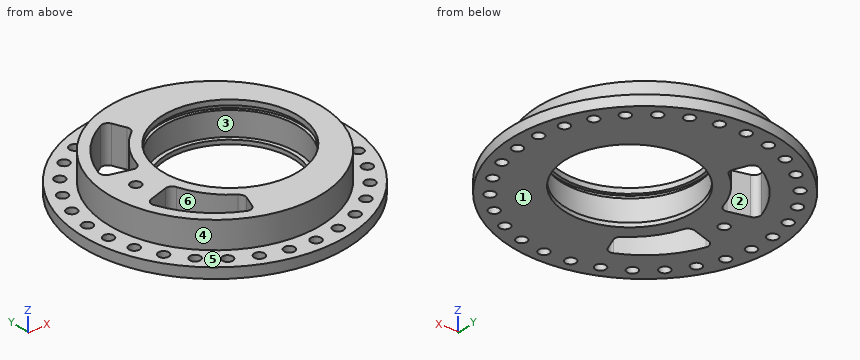
```python
from build123d import *

# Parameters (mm, degrees)
SKETCH1_R           = 63.5
BOSS_EXTRUDE1_DEPTH = 5
SKETCH2_R           = 51
BOSS_EXTRUDE2_DEPTH = 13
SKETCH3_R           = 32.5
CUT_EXTRUDE1_DEPTH  = 19
CUT_EXTRUDE9_START  = -2.5
SKETCH4_R           = 34
SKETCH4_R_2         = 32.5
CUT_EXTRUDE9_DEPTH  = 2
SKETCH6_R           = 32.5
SKETCH6_R_2         = 30.5
BOSS_EXTRUDE3_DEPTH = 2
SKETCH7_R           = 2.5
CUT_EXTRUDE10_DEPTH = 19
SKETCH9_R           = 2.5
CUT_EXTRUDE11_DEPTH = 19
CUT_EXTRUDE12_DEPTH = 19
FILLET1_R           = 3


with BuildPart() as part:
    # Sketch1 → Boss-Extrude1 (new body)
    with BuildSketch(Plane.XY):
        Circle(SKETCH1_R)
    extrude(amount=BOSS_EXTRUDE1_DEPTH)

    # Sketch2 → Boss-Extrude2 (add)
    with BuildSketch(Plane.XY.offset(5)):
        Circle(SKETCH2_R)
    extrude(amount=BOSS_EXTRUDE2_DEPTH)

    # Sketch3 → Cut-Extrude1 (cut, through all)
    with BuildSketch(Plane.XY.offset(18)):
        with Locations((7.5, 0)):
            Circle(SKETCH3_R)
    extrude(amount=-CUT_EXTRUDE1_DEPTH, mode=Mode.SUBTRACT)

    # Sketch4 → Cut-Extrude9 (cut)
    with BuildSketch(Plane.XY.offset(18).offset(CUT_EXTRUDE9_START)):
        with Locations((7.5, 0)):
            Circle(SKETCH4_R)
        with Locations((7.5, 0)):
            Circle(SKETCH4_R_2, mode=Mode.SUBTRACT)
    extrude(amount=-CUT_EXTRUDE9_DEPTH, mode=Mode.SUBTRACT)

    # Sketch6 → Boss-Extrude3 (add)
    with BuildSketch(Plane(origin=(0, 0, 0), x_dir=(-1, 0, 0), z_dir=(0, 0, -1))):
        with Locations((-7.5, 0)):
            Circle(SKETCH6_R)
        with Locations((-7.5, 0)):
            Circle(SKETCH6_R_2, mode=Mode.SUBTRACT)
    extrude(amount=-BOSS_EXTRUDE3_DEPTH)

    # Sketch7 → Cut-Extrude10 (cut, through all)
    with BuildSketch(Plane.XY.offset(18)):
        with Locations((0, 57.24)):
            Circle(SKETCH7_R)
        with Locations((11.900865182, 55.989168666)):
            Circle(SKETCH7_R)
        with Locations((23.28160545, 52.291341995)):
            Circle(SKETCH7_R)
        with Locations((33.644827841, 46.308132758)):
            Circle(SKETCH7_R)
        with Locations((42.53760981, 38.301035908)):
            Circle(SKETCH7_R)
        with Locations((49.571294113, 28.62)):
            Circle(SKETCH7_R)
        with Locations((54.438474993, 17.688132758)):
            Circle(SKETCH7_R)
        with Locations((56.926433291, 5.983209237)):
            Circle(SKETCH7_R)
        with Locations((56.926433291, -5.983209237)):
            Circle(SKETCH7_R)
        with Locations((54.438474993, -17.688132758)):
            Circle(SKETCH7_R)
        with Locations((49.571294113, -28.62)):
            Circle(SKETCH7_R)
        with Locations((42.53760981, -38.301035908)):
            Circle(SKETCH7_R)
        with Locations((33.644827841, -46.308132758)):
            Circle(SKETCH7_R)
        with Locations((23.28160545, -52.291341995)):
            Circle(SKETCH7_R)
        with Locations((11.900865182, -55.989168666)):
            Circle(SKETCH7_R)
        with Locations((0, -57.24)):
            Circle(SKETCH7_R)
        with Locations((-11.900865182, -55.989168666)):
            Circle(SKETCH7_R)
        with Locations((-23.28160545, -52.291341995)):
            Circle(SKETCH7_R)
        with Locations((-33.644827841, -46.308132758)):
            Circle(SKETCH7_R)
        with Locations((-42.53760981, -38.301035908)):
            Circle(SKETCH7_R)
        with Locations((-49.571294113, -28.62)):
            Circle(SKETCH7_R)
        with Locations((-54.438474993, -17.688132758)):
            Circle(SKETCH7_R)
        with Locations((-56.926433291, -5.983209237)):
            Circle(SKETCH7_R)
        with Locations((-56.926433291, 5.983209237)):
            Circle(SKETCH7_R)
        with Locations((-54.438474993, 17.688132758)):
            Circle(SKETCH7_R)
        with Locations((-49.571294113, 28.62)):
            Circle(SKETCH7_R)
        with Locations((-42.53760981, 38.301035908)):
            Circle(SKETCH7_R)
        with Locations((-33.644827841, 46.308132758)):
            Circle(SKETCH7_R)
        with Locations((-23.28160545, 52.291341995)):
            Circle(SKETCH7_R)
        with Locations((-11.900865182, 55.989168666)):
            Circle(SKETCH7_R)
    extrude(amount=-CUT_EXTRUDE10_DEPTH, mode=Mode.SUBTRACT)

    # Sketch9 → Cut-Extrude11 (cut, through all)
    with BuildSketch(Plane.XY.offset(18)):
        with Locations((-38.5, 0)):
            Circle(SKETCH9_R)
    extrude(amount=-CUT_EXTRUDE11_DEPTH, mode=Mode.SUBTRACT)

    # Sketch10 → Cut-Extrude12 (cut, through all)
    with BuildSketch(Plane.XY.offset(18)):
        with BuildLine():
            Line((-12.751630161, 31.561392172), (-17.231903297, 42.65045731))
            ThreePointArc((-17.231903297, 42.65045731), (-34.184661972, 30.780007893), (-44.218038013, 12.679318368))
            Line((-44.218038013, 12.679318368), (-29.062316979, 8.333485293))
            ThreePointArc((-29.062316979, 8.333485293), (-23.189412863, 21.550172577), (-12.751630161, 31.561392172))
        make_face()
        with BuildLine():
            Line((-12.751630161, -31.561392172), (-17.231903297, -42.65045731))
            ThreePointArc((-17.231903297, -42.65045731), (-34.184661972, -30.780007893), (-44.218038013, -12.679318368))
            Line((-44.218038013, -12.679318368), (-29.062316979, -8.333485293))
            ThreePointArc((-29.062316979, -8.333485293), (-23.189412863, -21.550172577), (-12.751630161, -31.561392172))
        make_face()
    extrude(amount=-CUT_EXTRUDE12_DEPTH, mode=Mode.SUBTRACT)

    # Fillet1
    fillet1_edges = [part.edges().sort_by_distance(p)[0] for p in [
        (-12.751630161, 31.561392172, 9),
        (-29.062316979, 8.333485293, 9),
        (-44.218038013, 12.679318368, 9),
        (-17.231903297, 42.65045731, 9),
        (-29.062316979, -8.333485293, 9),
        (-12.751630161, -31.561392172, 9),
        (-17.231903297, -42.65045731, 9),
        (-44.218038013, -12.679318368, 9),
    ]]
    fillet(fillet1_edges, radius=FILLET1_R)


solid = part.part
```
CAD build for the part. Positions are in the model's coordinates, mm. Face numbers are marked on the shaded views. A direction names the side the tool comes from. Round coordinates to 2 decimals unless told otherwise and drop trailing zeros. Order: outer loops, then holes, each group sorted by start corner. A loop starts at its lowest first (then second) coordinate and runs counter-clockwise, first axis right, second up. Notation, with made-up numbers: (77.5, 70) - (130.5, 70) arc R15 ccw to (130.5, 99) - close; hole circle Ø4 at (76.25, -34). An arc over 180 degrees is marked (long way). Answer in a Markdown table with one row per item. Add a question column.
(1) Band-saw the part on A-A on y = 0. List the corners of the cut face in (x, z), and give its area (3 significant figures).
(2) Drop flat-ended pins along their axis: pin 1 Ø2 at (y, z) = (-41, 11) entering from +X; pin 2 Ø8 at (x, y) = (42.54, 38.3) entering from +Z; pin 3 Ø4.5 at (x, y) = (11.9, -55.99) entering from +Z; pin 4 Ø3 at (x, z) = (-36.5, 12.5) entering from -Y. Give the stop position or say it passes through.
(3) 3-axis set-ups, long thin cutter, end or side, ignore diameter. For the marked faces 1 and 2: which of +Z, -Z, +X, -X, +Y, -Y reach the whole face in a straight line?
(4) Mould opens along Y. For the marked faces 3, 4, 5 and 6 say: +Y half, -Y half, draft (parallel to the pull), parting line (faces both ways), or undercut.
(5) Band-saw the part on B-B on x = 11. Count the separate pieces of the cut face and the enclosed holes in it, and give its area (3 significant figures).
(6) Band-saw the part on D-D on x = -38.5. List the corners of the cut face in (y, z), and give its area (3 significant figures).
(7) Band-saw the part on C-C on y = -24. List the corners of the cut face in (x, z), and give its area (3 significant figures).
(8) Probe L1, parallel to Y at x = -22, z = 13; L2, parallel to Y at x = -19, z = 7; L3, parallel to X at y = -17, z = 17.25. List the from-to ranges inside material, lowest first. Write a range as [from, to].
Data:
| question | item | result |
|---|---|---|
| 1 | outline | (-63.5, 0) - (-41, 0) - (-41, 18) - (-51, 18) - (-51, 5) - (-63.5, 5) - close; (-36, 0) - (-23, 0) - (-23, 2) - (-25, 2) - (-25, 13.5) - (-26.5, 13.5) - (-26.5, 15.5) - (-25, 15.5) - (-25, 18) - (-36, 18) - close; (38, 0) - (63.5, 0) - (63.5, 5) - (51, 5) - (51, 18) - (40, 18) - (40, 15.5) - (41.5, 15.5) - (41.5, 13.5) - (40, 13.5) - (40, 2) - (38, 2) - close |
| 1 | area | 703 mm^2 |
| 2 | pin 1 | stops at x = 31.64 |
| 2 | pin 2 | stops at z = 5 |
| 2 | pin 3 | passes through |
| 2 | pin 4 | stops at y = -37.09 |
| 3 | face 1 | -Z, +X, -X, +Y, -Y |
| 3 | face 2 | +Z, -Z |
| 4 | face 3 | undercut |
| 4 | face 4 | parting line |
| 4 | face 5 | draft |
| 4 | face 6 | undercut |
| 5 | separate pieces | 4 |
| 5 | enclosed holes | 0 |
| 5 | area | 712 mm^2 |
| 6 | outline | (-50.5, 0) - (-25.17, 0) - (-25.17, 18) - (-33.45, 18) - (-33.45, 5) - (-50.5, 5) - close; (-11.04, 0) - (-2.5, 0) - (-2.5, 18) - (-11.04, 18) - close; (2.5, 0) - (11.04, 0) - (11.04, 18) - (2.5, 18) - close; (25.17, 0) - (50.5, 0) - (50.5, 5) - (33.45, 5) - (33.45, 18) - (25.17, 18) - close |
| 6 | area | 776 mm^2 |
| 7 | outline | (-58.79, 0) - (-39.24, 0) - (-39.24, 18) - (-45, 18) - (-45, 5) - (-58.79, 5) - close; (-21.31, 0) - (-11.32, 0) - (-11.32, 2) - (-14.41, 2) - (-14.41, 13.5) - (-16.58, 13.5) - (-16.58, 15.5) - (-14.41, 15.5) - (-14.41, 18) - (-21.31, 18) - close; (26.32, 0) - (58.79, 0) - (58.79, 5) - (45, 5) - (45, 18) - (29.41, 18) - (29.41, 15.5) - (31.58, 15.5) - (31.58, 13.5) - (29.41, 13.5) - (29.41, 2) - (26.32, 2) - close |
| 7 | area | 650 mm^2 |
| 8 | L1 | y = [-46.01, -40.4], [-23.15, -13.64], [13.64, 23.15], [40.4, 46.01] |
| 8 | L2 | y = [-47.33, -41.64], [-26.53, -18.81], [18.81, 26.53], [41.64, 47.33] |
| 8 | L3 | x = [-48.08, -42.74], [-25.93, -20.2], [35.2, 48.08] |
